from build123d import *

# Parameters (mm, degrees)
F0_R     = 1.55
F0_W     = 6
F0_H     = 6
F0_W_2   = 8
F1_DEPTH = 6


with BuildPart() as f1:
    # F0 (on Front) → F1 (new body)
    with BuildSketch(Plane.XZ):
        with BuildLine():
            Line((290, 33.159883), (-290, 33.159883))
            ThreePointArc((-290, 33.159883), (-293.535534, 31.695417), (-295, 28.159883))
            Line((-295, 28.159883), (-295, -11.840117))
            ThreePointArc((-295, -11.840117), (-293.535534, -15.375651), (-290, -16.840117))
            Line((-290, -16.840117), (290, -16.840117))
            ThreePointArc((290, -16.840117), (293.535534, -15.375651), (295, -11.840117))
            Line((295, -11.840117), (295, 28.159883))
            ThreePointArc((295, 28.159883), (293.535534, 31.695417), (290, 33.159883))
        make_face()
        with Locations((-285, -9.340117)):
            Circle(F0_R, mode=Mode.SUBTRACT)
        with Locations((-260, -9.340117)):
            Rectangle(F0_W, F0_H, mode=Mode.SUBTRACT)
        with Locations((-245, -9.340117)):
            Rectangle(F0_W_2, F0_H, mode=Mode.SUBTRACT)
        with Locations((-230, -9.340117)):
            Rectangle(F0_W, F0_H, mode=Mode.SUBTRACT)
        with Locations((-185, -9.340117)):
            Circle(F0_R, mode=Mode.SUBTRACT)
        with Locations((-137.5, -9.304218)):
            Rectangle(F0_W, F0_H, mode=Mode.SUBTRACT)
        with Locations((-122.5, -9.304218)):
            Rectangle(F0_W_2, F0_H, mode=Mode.SUBTRACT)
        with Locations((-107.5, -9.304218)):
            Rectangle(F0_W, F0_H, mode=Mode.SUBTRACT)
        with Locations((-60, -9.340117)):
            Circle(F0_R, mode=Mode.SUBTRACT)
        with Locations((-15, -9.268318)):
            Rectangle(F0_W, F0_H, mode=Mode.SUBTRACT)
        with Locations((0, -9.268318)):
            Rectangle(F0_W_2, F0_H, mode=Mode.SUBTRACT)
        with Locations((15, -9.268318)):
            Rectangle(F0_W, F0_H, mode=Mode.SUBTRACT)
        with Locations((65, -9.340117)):
            Circle(F0_R, mode=Mode.SUBTRACT)
        with Locations((112.5, -9.304218)):
            Rectangle(F0_W, F0_H, mode=Mode.SUBTRACT)
        with Locations((127.5, -9.304218)):
            Rectangle(F0_W_2, F0_H, mode=Mode.SUBTRACT)
        with Locations((142.5, -9.304218)):
            Rectangle(F0_W, F0_H, mode=Mode.SUBTRACT)
        with Locations((190, -9.340117)):
            Circle(F0_R, mode=Mode.SUBTRACT)
        with Locations((240, -9.340117)):
            Rectangle(F0_W, F0_H, mode=Mode.SUBTRACT)
        with Locations((255, -9.340117)):
            Rectangle(F0_W_2, F0_H, mode=Mode.SUBTRACT)
        with Locations((270, -9.340117)):
            Rectangle(F0_W, F0_H, mode=Mode.SUBTRACT)
        with Locations((285, -9.340117)):
            Circle(F0_R, mode=Mode.SUBTRACT)
        with Locations((-285, 25.659883)):
            Circle(F0_R, mode=Mode.SUBTRACT)
        with Locations((-260, 25.659883)):
            Rectangle(F0_W, F0_H, mode=Mode.SUBTRACT)
        with Locations((-245, 25.659883)):
            Rectangle(F0_W_2, F0_H, mode=Mode.SUBTRACT)
        with Locations((-230, 25.659883)):
            Rectangle(F0_W, F0_H, mode=Mode.SUBTRACT)
        with Locations((-185, 25.659883)):
            Circle(F0_R, mode=Mode.SUBTRACT)
        with Locations((-137.5, 25.623984)):
            Rectangle(F0_W, F0_H, mode=Mode.SUBTRACT)
        with Locations((-122.5, 25.623984)):
            Rectangle(F0_W_2, F0_H, mode=Mode.SUBTRACT)
        with Locations((-107.5, 25.623984)):
            Rectangle(F0_W, F0_H, mode=Mode.SUBTRACT)
        with Locations((-60, 25.659883)):
            Circle(F0_R, mode=Mode.SUBTRACT)
        with Locations((-15, 25.588085)):
            Rectangle(F0_W, F0_H, mode=Mode.SUBTRACT)
        with BuildLine():
            ThreePointArc((-280, 13.159883), (-278.535534, 16.695417), (-275, 18.159883))
            Line((-275, 18.159883), (275, 18.159883))
            ThreePointArc((275, 18.159883), (278.535534, 16.695417), (280, 13.159883))
            Line((280, 13.159883), (280, 3.159883))
            ThreePointArc((280, 3.159883), (278.535534, -0.375651), (275, -1.840117))
            Line((275, -1.840117), (-275, -1.840117))
            ThreePointArc((-275, -1.840117), (-278.535534, -0.375651), (-280, 3.159883))
            Line((-280, 3.159883), (-280, 13.159883))
        make_face(mode=Mode.SUBTRACT)
        with Locations((0, 25.588085)):
            Rectangle(F0_W_2, F0_H, mode=Mode.SUBTRACT)
        with Locations((15, 25.588085)):
            Rectangle(F0_W, F0_H, mode=Mode.SUBTRACT)
        with Locations((65, 25.659883)):
            Circle(F0_R, mode=Mode.SUBTRACT)
        with Locations((112.5, 25.623984)):
            Rectangle(F0_W, F0_H, mode=Mode.SUBTRACT)
        with Locations((127.5, 25.623984)):
            Rectangle(F0_W_2, F0_H, mode=Mode.SUBTRACT)
        with Locations((142.5, 25.623984)):
            Rectangle(F0_W, F0_H, mode=Mode.SUBTRACT)
        with Locations((190, 25.659883)):
            Circle(F0_R, mode=Mode.SUBTRACT)
        with Locations((240, 25.659883)):
            Rectangle(F0_W, F0_H, mode=Mode.SUBTRACT)
        with Locations((255, 25.659883)):
            Rectangle(F0_W_2, F0_H, mode=Mode.SUBTRACT)
        with Locations((270, 25.659883)):
            Rectangle(F0_W, F0_H, mode=Mode.SUBTRACT)
        with Locations((285, 25.659883)):
            Circle(F0_R, mode=Mode.SUBTRACT)
    extrude(amount=F1_DEPTH)


solid = f1.part
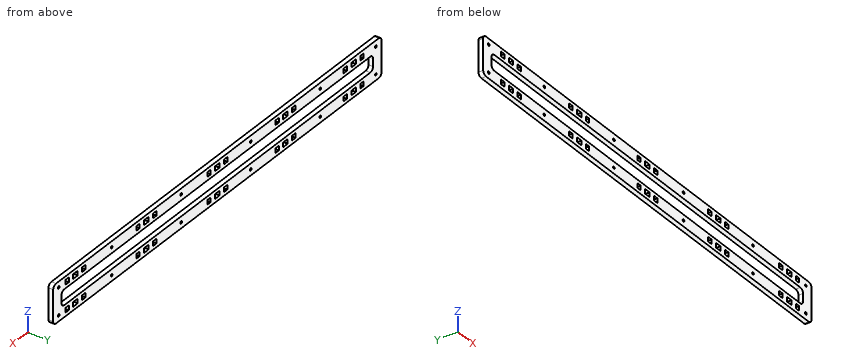
Work out the finished part from the listing and answer in its coordinate system (mm). Give positions to 0.01 mm unless a question says otherwise; leave off trailing zeros. Order: outer loops, then holes, each group sorted by start corner. A loop starts at its lowest first (then second) coordinate and runs counter-clockwise, first axis right, second up. Notation, with made-up numbers: (76, 21.25) -> (96, 21.25) arc R21 cw to (96, 55.25) -> close; hole circle Ø5 at (45.5, -13.75). An arc over 180 degrees is marked (long way). Answer as a JSON object with one key per item and string values. Group by question number.
1. Consider line 1 along Z through (x, y) = (-185, -2.55); line 2 along Z through (x, y) = (-2, -4.9); line 3 along X through (y, z) = (-3, 10). Determine where each line is inside the solid, lowest interval first. Write a range as [from, to].
2. Section A-A on x = 24 is taken. Determine the outline of the cut face in (y, z), plus the area to 3 significant figures.
3. Section B-B on y = -2.7 is taken. Count the separate pieces of the cut face and the enclosed holes in it, plus the area to 3 significant figures.
Result sheet:
{
 "1": {"line 1": "z = [-16.84, -10.89], [-7.79, -1.84], [18.16, 24.11], [27.21, 33.16]", "line 2": "z = [-16.84, -12.27], [-6.27, -1.84], [18.16, 22.59], [28.59, 33.16]", "line 3": "x = [-295, -280], [280, 295]"},
 "2": {"outline": "(-6, -16.84) -> (0, -16.84) -> (0, -1.84) -> (-6, -1.84) -> close; (-6, 18.16) -> (0, 18.16) -> (0, 33.16) -> (-6, 33.16) -> close", "area": "180 mm^2"},
 "3": {"separate pieces": "1", "enclosed holes": "43", "area": "17,000 mm^2"}
}
